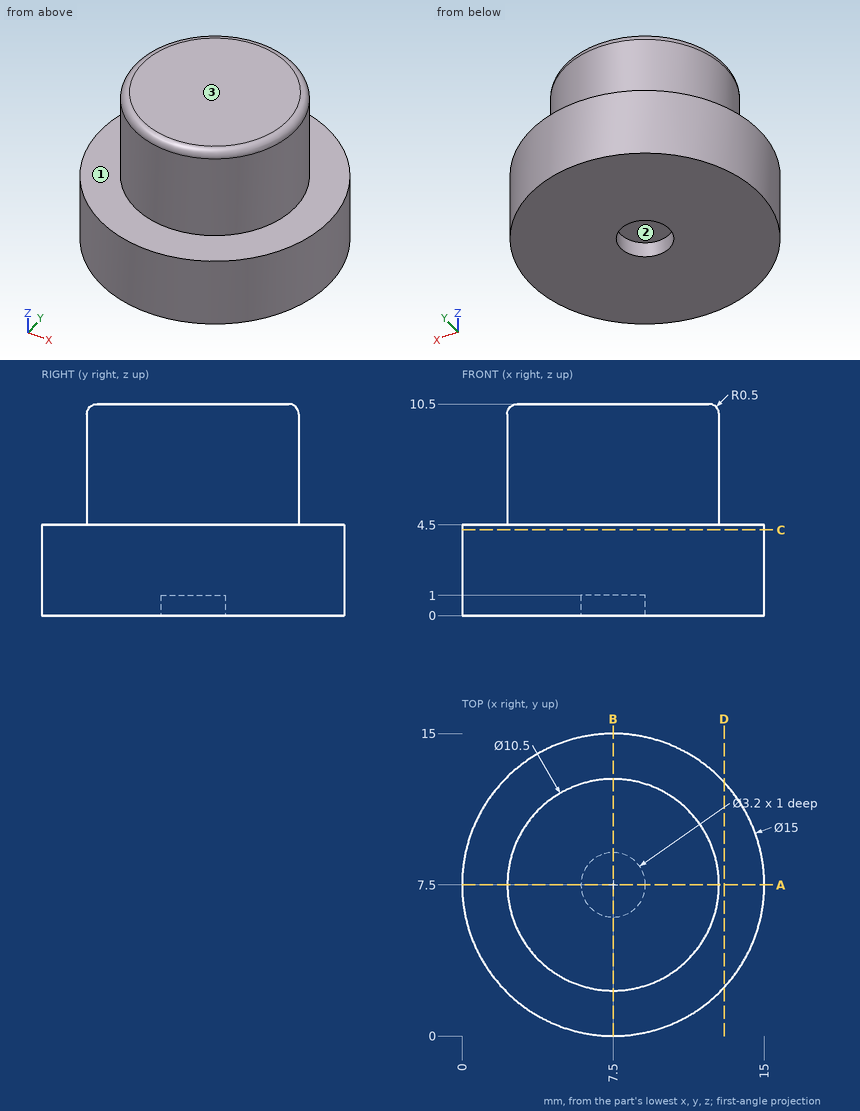
For this review, use the dimensioned drawing (mm, ordinates from the lowest corner) and the shaded views. A direction names the side the tool comes from. Coordinates: 2 decimals unless noted, no trailing zeros. Loops run counter-clockwise (first coordinate to the right, second up) from the corner with the lowest first, then second, coordinate; pieces in that order, holes last. Notation, with made-up numbers: (-30.75, -26) - (15.25, -26) arc R21 cw to (15.25, -4) - close; hole circle Ø8 at (57.25, -17.75). An arc over 180 degrees is marked (long way). Use CSV: the item, a comma, the result in double quotes. Start each with the question number.
1) Consider section C-C on z = 4.25. Write out the cut boundary in (x, y).
2) Wall thickness on L1, parallel to Y at x = 7.5, z = 0.25; L2, parallel to Z at x = 13.25, y = 6.5; L3, parallel to Y at x = 3, z = 6.25: over which ranges is each line inside the solid? List them lowest first. Write a range as from..to.
3) Tool access review of the marked faces 1, 2 and 3: name each direction out of +Z, -Z, +X, -X, +Y, -Y from which nothing blocks a thin tool from reaching the whole face with its end or side.
4) For pin 1 Ø1.5 at (x, y) = (6.5, 1.5) entering from +Z; pin 2 Ø1.5 at (x, z) = (9.5, 5.5) entering from +Y; pin 3 Ø6 at (y, z) = (3, 6) entering from +X, all flat-tipped, find the tip position at first contact; note any pin that passes through.
5) Consider section A-A on y = 7.5. Write out the cut boundary in (x, z), then the cut area to 3 significant figures.
6) Consider section D-D on x = 13. Write out the cut boundary in (y, z), then the cut area to 3 significant figures.
Geometry says:
1,outline,"circle Ø15 at (7.5, 7.5)"
2,L1,"0..5.9, 9.1..15"
2,L2,"0..4.5"
2,L3,"4.8..10.2"
3,face 1,"+Z"
3,face 2,"-Z"
3,face 3,"+Z, +X, -X, +Y, -Y"
4,pin 1,"z = 4.5"
4,pin 2,"y = 12.6"
4,pin 3,"x = 14.75"
5,outline,"(0, 0) - (5.9, 0) - (5.9, 1) - (9.1, 1) - (9.1, 0) - (15, 0) - (15, 4.5) - (12.75, 4.5) - (12.75, 10) arc R0.5 ccw to (12.25, 10.5) - (2.75, 10.5) arc R0.5 ccw to (2.25, 10) - (2.25, 4.5) - (0, 4.5) - close"
5,area,"127 mm^2"
6,outline,"(2.4, 0) - (12.6, 0) - (12.6, 4.5) - (2.4, 4.5) - close"
6,area,"45.9 mm^2"
